Drawing for the job (mm, zero at the part's lowest x, y, z). Give positions to 0.01 mm unless a question says otherwise; leave off trailing zeros. Order: outer loops, then holes, each group sorted by start corner. A loop starts at its lowest first (then second) coordinate and runs counter-clockwise, first axis right, second up. Notation, with made-up numbers: (-18.75, -40) - (34.25, -40) arc R29 cw to (34.25, -7) - close; hole circle Ø10 at (63, 29.25). An arc over 180 degrees is marked (long way). Write each question's results on one line, items separated by ' | '. Start each with the question number.
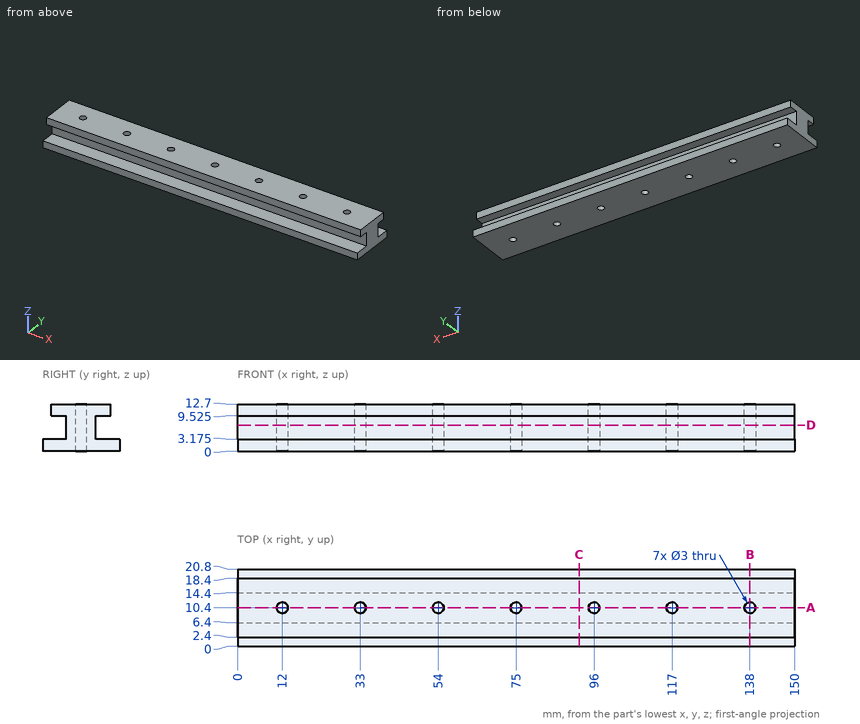
Item 1: Cut at A-A, the plane y = 10.4. Count the separate pieces of the cut face and the enclosed holes in it, then the cut area to 3 significant figures.
Item 2: Cut at D-D, the plane z = 7. List the corners of the cut face in (x, y).
Item 3: Probe line 1 along Z through (x, y) = (92.5, 17) (3 decimals); line 2 along Z through (x, y) = (99, 19.75) (3 decimals); line 3 along Y through (x, z) = (11.5, 4.5). List the from-to ranges inside material, lowest first. Write a range as from..to.
Item 4: Cut at C-C, the plane x = 92. List the corners of the cut face in (y, z) (3 decimals), then the cut area to 3 significant figures.
Item 5: Flat gauge pins, fed straight in: pin 1 Ø2 at (x, z) = (111.5, 6.5) entering from -Y; pin 2 Ø6 at (x, z) = (83.5, 8) entering from +Y; pin 3 Ø1.6 at (x, z) = (59, 10.5) entering from -Y. Where does each tip first touch, or does it go through?
Item 6: Cut at B-B, the plane x = 138. List the corners of the cut face in (y, z) (3 decimals), then the cut area to 3 significant figures.
Values found:
1) separate pieces: 8 | enclosed holes: 0 | area: 1,640 mm2
2) outline: (0, 6.4) - (150, 6.4) - (150, 14.4) - (0, 14.4) - close; hole circle Ø3 at (12, 10.4); hole circle Ø3 at (33, 10.4); hole circle Ø3 at (54, 10.4); hole circle Ø3 at (75, 10.4); hole circle Ø3 at (96, 10.4); hole circle Ø3 at (117, 10.4); hole circle Ø3 at (138, 10.4)
3) line 1: z = 0..3.175, 9.525..12.7 | line 2: z = 0..3.175 | line 3: y = 6.4..8.99, 11.81..14.4
4) outline: (0, 0) - (20.8, 0) - (20.8, 3.175) - (14.4, 3.175) - (14.4, 9.525) - (18.4, 9.525) - (18.4, 12.7) - (2.4, 12.7) - (2.4, 9.525) - (6.4, 9.525) - (6.4, 3.175) - (0, 3.175) - close | area: 168 mm2
5) pin 1: stops at y = 6.4 | pin 2: stops at y = 18.4 | pin 3: stops at y = 2.4
6) outline: (0, 0) - (8.9, 0) - (8.9, 12.7) - (2.4, 12.7) - (2.4, 9.525) - (6.4, 9.525) - (6.4, 3.175) - (0, 3.175) - close; (11.9, 0) - (20.8, 0) - (20.8, 3.175) - (14.4, 3.175) - (14.4, 9.525) - (18.4, 9.525) - (18.4, 12.7) - (11.9, 12.7) - close | area: 130 mm2
